```python
from build123d import *

# Parameters (mm, degrees)
F0_W     = 406.4
F0_H     = 381
F1_DEPTH = 6.35
F3_DEPTH = 52.07
F4_W     = 19.6954607964
F4_H     = 38.0410514772
F5_DEPTH = 25.4
F7_DEPTH = 25.4
F8_W     = 266.1207329154
F8_H     = 104.222646597
F8_W_2   = 253.4207329154
F8_H_2   = 91.522646597
F9_DEPTH = 6.35


with BuildPart() as f1:
    # F0 (on Top) → F1 (new body)
    with BuildSketch(Plane.XY):
        with Locations((-7.9120187303, 477.383510977)):
            Rectangle(F0_W, F0_H)
    extrude(amount=-F1_DEPTH)

    # F2 (on face) → F3 (join)
    with BuildSketch(Plane.XY):
        Polygon((-89.1544180155, 661.533510977), (-89.1544180155, 534.533510977), (-28.623964709, 534.533510977), (-28.623964709, 490.0471397191), (15.826035291, 490.0471397191), (15.826035291, 413.8471397191), (-104.9383804202, 413.8471397191), (-104.9383804202, 309.6244931221), (161.1823524952, 309.6244931221), (161.1823524952, 413.8471397191), (48.055235368, 413.8471397191), (48.055235368, 490.0471397191), (92.505235368, 490.0471397191), (92.505235368, 585.333510977), (92.505235368, 610.733510977), (92.505235368, 617.083510977), (-19.8705563486, 617.083510977), (-19.8705563486, 661.533510977), align=None)
        Polygon((22.176035291, 585.333510977), (-28.623964709, 585.333510977), (-28.623964709, 540.883510977), (-82.8044180155, 540.883510977), (-82.8044180155, 655.183510977), (-28.623964709, 655.183510977), (-28.623964709, 610.733510977), (86.155235368, 610.733510977), (86.155235368, 585.333510977), (41.705235368, 585.333510977), (41.705235368, 578.983510977), (86.155235368, 578.983510977), (86.155235368, 496.4115063727), (41.705235368, 496.4115063727), (41.705235368, 490.0471397191), (41.705235368, 407.4971397191), (154.8323524952, 407.4971397191), (154.8323524952, 315.9744931221), (-98.5883804202, 315.9744931221), (-98.5883804202, 407.4971397191), (22.176035291, 407.4971397191), (22.176035291, 490.0471397191), (22.176035291, 496.3971397191), (-22.273964709, 496.3971397191), (-22.273964709, 578.983510977), (22.176035291, 578.983510977), align=None, mode=Mode.SUBTRACT)
    extrude(amount=F3_DEPTH)

    # F4 (on face) → F5 (cut)
    with BuildSketch(Plane(origin=(-89.1544180155, 0, 0), x_dir=(0, -1, 0), z_dir=(-1, 0, 0))):
        with Locations((-620.421141386, 19.0205257386)):
            Rectangle(F4_W, F4_H)
    extrude(amount=-F5_DEPTH, mode=Mode.SUBTRACT)

    # F6 (on face) → F7 (join)
    with BuildSketch(Plane.XZ.offset(-407.4971397191)):
        Polygon((41.705235368, 5.08), (41.705235368, 0), (110.285235368, 0), (110.285235368, 45.72), (102.665235368, 45.72), (102.665235368, 40.64), (95.045235368, 40.64), (95.045235368, 35.56), (87.425235368, 35.56), (87.425235368, 30.48), (79.805235368, 30.48), (79.805235368, 25.4), (72.185235368, 25.4), (72.185235368, 20.32), (64.565235368, 20.32), (64.565235368, 15.24), (56.945235368, 15.24), (56.945235368, 10.16), (49.325235368, 10.16), (49.325235368, 5.08), align=None)
    extrude(amount=F7_DEPTH)

    # F8 (on face) → F9 (join)
    with BuildSketch(Plane.XY.offset(52.07)):
        with Locations((28.1219860375, 361.7358164206)):
            Rectangle(F8_W, F8_H)
        with Locations((28.1219860375, 361.7358164206)):
            Rectangle(F8_W_2, F8_H_2, mode=Mode.SUBTRACT)
    extrude(amount=-F9_DEPTH)


solid = f1.part
```
CAD build for the part. Positions are in the model's coordinates, mm. A direction names the side the tool comes from. Round coordinates to 2 decimals unless told otherwise and drop trailing zeros. Loops run counter-clockwise (first coordinate to the right, second up) from the corner with the lowest first, then second, coordinate; pieces in that order, holes last. Notation, with made-up numbers: M 22.5,-28 L 76.5,-28 A24 ccw 76.5,-1 Z; hole C 51,-12.75 d5. An arc over 180 degrees is marked long. Use a Markdown table: item, result. Add a question column.
(1) Cut at C-C (y = 563.5). Give the cut face in (x, z).
(2) Flat gauge pins, fed straight in: pin 1 (1.5 mm diameter, centred on y = 396.5, z = 33, fed in from -X); pin 2 (10 mm diameter, centred on x = -103.5, z = 18, fed in from +Y); pin 3 (22 mm diameter, centred on x = 4, z = 22, fed in from -Y). Where does each tip first touch, or does it go through?
(3) Cut at B-B (x = -160.5). Give the cut face in (y, z), and give its area (3 significant figures).
(4) Cut at A-A (y = 321). Give the cut face in (x, z), and give its area (3 significant figures).
(5) Pull direction Y, two halves, no side cores. Call faces 4 (the face through (161.182, 361, 26)), 5 (the face through (48.055, 451, 26)): +Y half, -Y half, draft (parallel to the pull), parting line (faces both ways), or undercut.
(6) Which spindle directions (+Z, -Z, +X, -X, +Y, -Y) get a long thin tool onto all of the face, cutting with end or side? Do faces 1 (the face through (64, 578.984, 26)), 2 (the face through (-7, 490.047, 26)), 3 (the face through (92.505, 553, 26)). Say none if no direction does.
(7) Drill centre lines: line 1 (Y direction, x = 77.5, z = 42.5); line 2 (X direction, y = 382.5, z = 41.5); line 3 (X direction, y = 398, z = 18.5). Where is each one in solid material? Low to high.
Geometry says:
| question | item | result |
|---|---|---|
| 1 | outline | M -211.11,-6.35 L 195.29,-6.35 L 195.29,0 L 92.51,0 L 92.51,52.07 L 86.16,52.07 L 86.16,0 L -22.27,0 L -22.27,52.07 L -28.62,52.07 L -28.62,0 L -82.8,0 L -82.8,52.07 L -89.15,52.07 L -89.15,0 L -211.11,0 Z |
| 2 | pin 1 | stops at x = -104.94 |
| 2 | pin 2 | stops at y = 413.85 |
| 2 | pin 3 | stops at y = 309.62 |
| 3 | outline | M 286.88,-6.35 L 667.88,-6.35 L 667.88,0 L 286.88,0 Z |
| 3 | area | 2,420 mm² |
| 4 | outline | M -211.11,-6.35 L 195.29,-6.35 L 195.29,0 L 161.18,0 L 161.18,52.07 L 154.83,52.07 L 154.83,0 L -98.59,0 L -98.59,52.07 L -104.94,52.07 L -104.94,0 L -211.11,0 Z |
| 4 | area | 3,240 mm² |
| 5 | face 4 | draft |
| 5 | face 5 | undercut |
| 6 | face 1 | +Z |
| 6 | face 2 | +Z, -X |
| 6 | face 3 | +Z, +X, +Y |
| 7 | line 1 | y = 309.62 to 315.97, 407.5 to 413.85, 490.05 to 496.41, 578.98 to 585.33, 610.73 to 617.08 |
| 7 | line 2 | x = -104.94 to -98.59, 102.67 to 110.29, 154.83 to 161.18 |
| 7 | line 3 | x = -104.94 to -98.59, 64.57 to 110.29, 154.83 to 161.18 |
